The figure shows three views and two pictorial views of one solid part (mm, origin at its lowest corner). Answer the questions. A direction names the side the tool comes from. Coordinates: 2 decimals unless noted, no trailing zeros. Order: outer loops, then holes, each group sorted by start corner. A loop starts at its lowest first (then second) coordinate and runs counter-clockwise, first axis right, second up. Notation, with made-up numbers: (17, 12) -> (68, 12) arc R23 ccw to (68, 40) -> close; hole circle Ø3 at (-32.75, 75). An arc over 180 degrees is marked (long way). Write item = value, one per line. Start each with the question number.
Q1. Flat-ended cylindrical pins translate along their axes: pin 1 (1.6 mm diameter, centred on x = 3.5, y = 1.5, fed in from -Z); pin 2 (1.1 mm diameter, centred on x = 3.5, y = 1.5, fed in from +Z); pin 3 (0.7 mm diameter, centred on x = 3.5, z = 2, fed in from +Y). Find the tip coordinate at first contact, or state that the pin passes through.
Q2. The part is cut by section D-D, the plane y = 1.6. Count the separate pieces of the cut face and the enclosed holes in it, plus the area to 3 significant figures.
Q3. The part is cut by section B-B, the plane x = 1.5. Determine the outline of the cut face in (y, z).
Q4. The part is cut by section C-C, the plane y = 0.6. Determine the outline of the cut face in (x, z) (1 decimal).
Q5. Straight lines are drawn through the part: L1, parallel to Y at x = 1.5, z = 2.6; L2, parallel to X at y = 1.3, z = 2; L3, parallel to X at y = 0.65, z = 1.8 (1 decimal). For each, find the intervals that lie inside material, in ascending order. Write a range as from..to.
Q6. For a pull along X with two mould halves and no side action, classify the marked faces 1, 2 and 3 as +X half, -X half, draft (parallel to the pull), parting line (faces both ways), or undercut.
Q7. Which of the six approach directions +Z, -Z, +X, -X, +Y, -Y give full straight-line access (tool end or side, diameter ignored) to the marked faces 4, 5 and 6?
Q8. The part is cut by section A-A, the plane z = 2. Determine the outline of the cut face in (x, y).
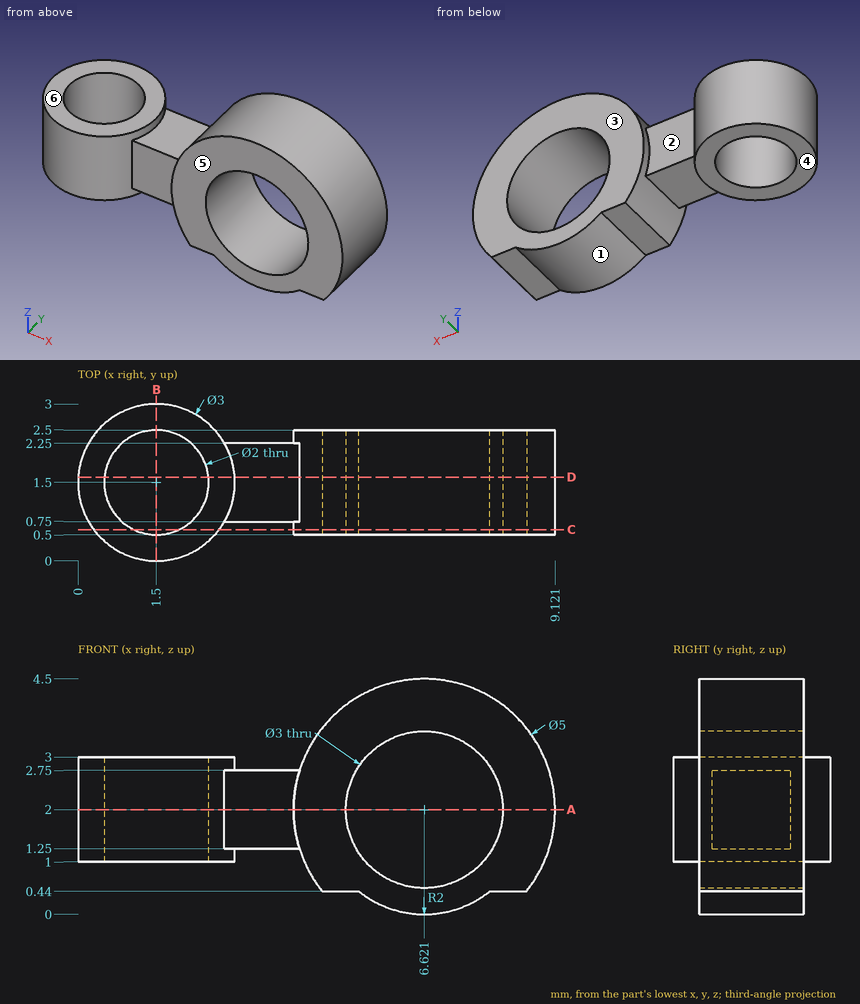
Model answer:
q1.pin_1 = 1
q1.pin_2 = 3
q1.pin_3 = 2.25
q2.separate_pieces = 2
q2.enclosed_holes = 1
q2.area = 14.5 mm2
q3.outline = (0, 1) -> (0.5, 1) -> (0.5, 3) -> (0, 3) -> close; (2.5, 1) -> (3, 1) -> (3, 3) -> (2.5, 3) -> close
q4.outline = (0.3, 1) -> (1.1, 1) -> (1.1, 3) -> (0.3, 3) -> close; (1.9, 1) -> (2.7, 1) -> (2.7, 3) -> (1.9, 3) -> close; (4.7, 0.4) -> (5.4, 0.4) arc R2 ccw to (7.9, 0.4) -> (8.6, 0.4) arc R2.5 ccw (long way) to start; hole circle Ø3 at (6.6, 2)
q5.L1 = 0..0.5, 2.5..3
q5.L2 = 0.01..0.52, 2.48..5.12, 8.12..9.12
q5.L3 = 0.3..1, 2..2.7, 4.1..5.1, 8.1..9.1
q6.face_1 = parting line
q6.face_2 = undercut
q6.face_3 = draft
q7.face_4 = -Z, -X, +Y, -Y
q7.face_5 = +Z, -Z, +X, -Y
q7.face_6 = +Z, -X, +Y, -Y
q8.outline = (2.8, 0.75) -> (4.12, 0.75) -> (4.12, 0.5) -> (5.12, 0.5) -> (5.12, 2.5) -> (4.12, 2.5) -> (4.12, 2.25) -> (2.8, 2.25) arc R1.5 ccw (long way) to start; (8.12, 0.5) -> (9.12, 0.5) -> (9.12, 2.5) -> (8.12, 2.5) -> close; hole circle Ø2 at (1.5, 1.5)
